```python
from build123d import *

# Parameters (mm, degrees)
F0_W         = 40
F0_H         = 70
F1_DEPTH     = 7
F2_R         = 5
F3_R         = 2
F4_DEPTH     = 5
F5_T1_DEPTH  = 60
F5_T3_DEPTH  = 30
F5_T6_ANGLE  = 90
F5_T8_ANGLE  = 90
F5_T10_ANGLE = 90
F5_T12_ANGLE = 90
F5_T14_ANGLE = 90
F5_T16_ANGLE = 90
F5_T18_ANGLE = 90
F5_T20_ANGLE = 90
F6_R         = 4
F7_DEPTH     = 0.3
F8_R         = 0.2
F9_W         = 12.4906748533
F9_H         = 1.2735207565
F10_DEPTH    = 1


# Not quite as in the source:
# - a fillet or chamfer that OpenCascade refuses, or shapes differently, is made with other operations: its cross-section is extruded or revolved along the edge and cut away or added


with BuildPart() as f1:
    # F0 (on Top) → F1 (new body)
    with BuildSketch(Plane.XY):
        with Locations((20, 35)):
            Rectangle(F0_W, F0_H)
    extrude(amount=F1_DEPTH)

    # F2
    f2_edges = [f1.edges().sort_by_distance(p)[0] for p in [
        (40, 0, 3.5),
        (0, 0, 3.5),
        (40, 70, 3.5),
        (0, 70, 3.5),
    ]]
    fillet(f2_edges, radius=F2_R)

    # F3 (on face) → F4 (cut)
    with BuildSketch(Plane(origin=(0, 70, 0), x_dir=(-1, 0, 0), z_dir=(0, 1, 0))):
        with Locations((-30.8697689325, 3.5)):
            Circle(F3_R)
    extrude(amount=-F4_DEPTH, mode=Mode.SUBTRACT)

    # F5: fillet of radius 2 on 16 edges, made by hand

    # F5_s2 → F5_t1 (cut)
    with BuildSketch(Plane.XZ.offset(-65)):
        with BuildLine():
            ThreePointArc((0, 5), (0.5857864376, 6.4142135624), (2, 7))
            Line((2, 7), (0, 7))
            Line((0, 7), (0, 5))
        make_face()
        with BuildLine():
            ThreePointArc((38, 7), (39.4142135624, 6.4142135624), (40, 5))
            Line((40, 5), (40, 7))
            Line((40, 7), (38, 7))
        make_face()
        with BuildLine():
            ThreePointArc((0, 2), (0.5857864376, 0.5857864376), (2, 0))
            Line((2, 0), (0, 0))
            Line((0, 0), (0, 2))
        make_face()
        with BuildLine():
            ThreePointArc((38, 0), (39.4142135624, 0.5857864376), (40, 2))
            Line((40, 2), (40, 0))
            Line((40, 0), (38, 0))
        make_face()
    extrude(amount=F5_T1_DEPTH, mode=Mode.SUBTRACT)

    # F5_s4 → F5_t3 (cut)
    with BuildSketch(Plane.YZ.offset(5)):
        with BuildLine():
            ThreePointArc((68, 7), (69.4142135624, 6.4142135624), (70, 5))
            Line((70, 5), (70, 7))
            Line((70, 7), (68, 7))
        make_face()
        with BuildLine():
            ThreePointArc((2, 7), (0.5857864376, 6.4142135624), (0, 5))
            Line((0, 5), (0, 7))
            Line((0, 7), (2, 7))
        make_face()
        with BuildLine():
            ThreePointArc((68, 0), (69.4142135624, 0.5857864376), (70, 2))
            Line((70, 2), (70, 0))
            Line((70, 0), (68, 0))
        make_face()
        with BuildLine():
            ThreePointArc((2, 0), (0.5857864376, 0.5857864376), (0, 2))
            Line((0, 2), (0, 0))
            Line((0, 0), (2, 0))
        make_face()
    extrude(amount=F5_T3_DEPTH, mode=Mode.SUBTRACT)

    # F5_s5 → F5_t6 (revolve, cut)
    with BuildSketch(Plane.XZ.offset(-65)):
        with BuildLine():
            ThreePointArc((0, 5), (0.5857864376, 6.4142135624), (2, 7))
            Line((2, 7), (0, 7))
            Line((0, 7), (0, 5))
        make_face()
    revolve(axis=Axis((5, 65, 7), (0, 0, -1)), revolution_arc=F5_T6_ANGLE, mode=Mode.SUBTRACT)

    # F5_s7 → F5_t8 (revolve, cut)
    with BuildSketch(Plane.XZ.offset(-5)):
        with BuildLine():
            ThreePointArc((0, 5), (0.5857864376, 6.4142135624), (2, 7))
            Line((2, 7), (0, 7))
            Line((0, 7), (0, 5))
        make_face()
    revolve(axis=Axis((5, 5, 7), (0, 0, 1)), revolution_arc=F5_T8_ANGLE, mode=Mode.SUBTRACT)

    # F5_s9 → F5_t10 (revolve, cut)
    with BuildSketch(Plane.XZ.offset(-65)):
        with BuildLine():
            ThreePointArc((38, 7), (39.4142135624, 6.4142135624), (40, 5))
            Line((40, 5), (40, 7))
            Line((40, 7), (38, 7))
        make_face()
    revolve(axis=Axis((35, 65, 7), (0, 0, 1)), revolution_arc=F5_T10_ANGLE, mode=Mode.SUBTRACT)

    # F5_s11 → F5_t12 (revolve, cut)
    with BuildSketch(Plane.YZ.offset(35)):
        with BuildLine():
            ThreePointArc((2, 7), (0.5857864376, 6.4142135624), (0, 5))
            Line((0, 5), (0, 7))
            Line((0, 7), (2, 7))
        make_face()
    revolve(axis=Axis((35, 5, 7), (0, 0, 1)), revolution_arc=F5_T12_ANGLE, mode=Mode.SUBTRACT)

    # F5_s13 → F5_t14 (revolve, cut)
    with BuildSketch(Plane.XZ.offset(-65)):
        with BuildLine():
            ThreePointArc((2, 0), (0.5857864376, 0.5857864376), (0, 2))
            Line((0, 2), (0, 0))
            Line((0, 0), (2, 0))
        make_face()
    revolve(axis=Axis((5, 65, 0), (0, 0, -1)), revolution_arc=F5_T14_ANGLE, mode=Mode.SUBTRACT)

    # F5_s15 → F5_t16 (revolve, cut)
    with BuildSketch(Plane.XZ.offset(-5)):
        with BuildLine():
            ThreePointArc((2, 0), (0.5857864376, 0.5857864376), (0, 2))
            Line((0, 2), (0, 0))
            Line((0, 0), (2, 0))
        make_face()
    revolve(axis=Axis((5, 5, 0), (0, 0, 1)), revolution_arc=F5_T16_ANGLE, mode=Mode.SUBTRACT)

    # F5_s17 → F5_t18 (revolve, cut)
    with BuildSketch(Plane.XZ.offset(-65)):
        with BuildLine():
            ThreePointArc((38, 0), (39.4142135624, 0.5857864376), (40, 2))
            Line((40, 2), (40, 0))
            Line((40, 0), (38, 0))
        make_face()
    revolve(axis=Axis((35, 65, 0), (0, 0, 1)), revolution_arc=F5_T18_ANGLE, mode=Mode.SUBTRACT)

    # F5_s19 → F5_t20 (revolve, cut)
    with BuildSketch(Plane.YZ.offset(35)):
        with BuildLine():
            ThreePointArc((2, 0), (0.5857864376, 0.5857864376), (0, 2))
            Line((0, 2), (0, 0))
            Line((0, 0), (2, 0))
        make_face()
    revolve(axis=Axis((35, 5, 0), (0, 0, 1)), revolution_arc=F5_T20_ANGLE, mode=Mode.SUBTRACT)

    # F6 (on face) → F7 (cut)
    with BuildSketch(Plane.XY.offset(7)):
        with Locations((19.5677466691, 10.9801534563)):
            Circle(F6_R)
    extrude(amount=-F7_DEPTH, mode=Mode.SUBTRACT)

    # F8
    f8_edges = [f1.edges().sort_by_distance(p)[0] for p in [
        (15.567747, 10.980153, 7),
        (2.87868, 67.12132, 7),
        (2, 35, 7),
        (20, 68, 7),
        (2.87868, 2.87868, 7),
        (37.12132, 67.12132, 7),
        (20, 2, 7),
        (38, 35, 7),
        (37.12132, 2.87868, 7),
    ]]
    fillet(f8_edges, radius=F8_R)

    # F9 (on face) → F10 (cut)
    with BuildSketch(Plane.XZ):
        with Locations((20.2241037041, 3.5419908818)):
            Rectangle(F9_W, F9_H)
    extrude(amount=-F10_DEPTH, mode=Mode.SUBTRACT)


solid = f1.part
```
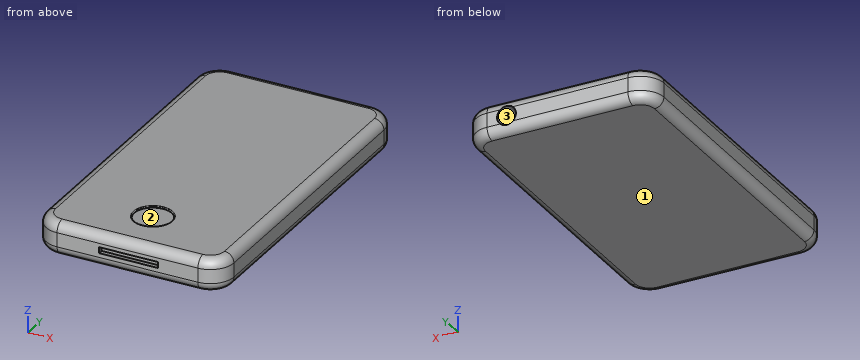
Geometry check sheet. Reference: the model listing, model coordinates, mm. Face numbers are marked on the shaded views. Coordinates: 2 decimals unless noted, no trailing zeros.
Item 1: Go/stop test with flat-tipped pins: pin 1 Ø0.5 at (y, z) = (0.5, 3.5) entering from +X; pin 2 Ø2.5 at (x, y) = (21.5, 12.5) entering from +Z; pin 3 Ø0.5 at (x, y) = (22, 0.5) entering from +Z. Record where each tip stops, or that it passes through.
Item 2: Thickness scan on line 1 (Y direction, x = 16, z = 4); line 2 (X direction, y = 11.5, z = 1.75); line 3 (X direction, y = 68.55, z = 3.5). Record the ranges inside material, lowest first.
Item 3: Release check for a two-part mould opening along X. For the marked faces 1, 2 and 3 record: released by +X, released by -X, zero draft, split by the parting line, or undercut.
Check result:
1. pin 1: stops at x = 37.63
1. pin 2: stops at z = 6.7
1. pin 3: stops at z = 6.56
2. line 1: y = 1 to 70
2. line 2: x = 0.02 to 39.98
2. line 3: x = 1.48 to 28.87, 32.87 to 38.52
3. face 1: zero draft
3. face 2: undercut
3. face 3: undercut
